Read the model definition and answer for the solid it produces. Units are mm, in the model's axes. Face numbers are marked on the shaded views. A direction names the side the tool comes from. Round coordinates to 2 decimals unless told otherwise and drop trailing zeros. Write each loop counter-clockwise with the first axis right and the second up, starting at its lowest first coordinate (ties: lowest second). Pieces come first, ordered by that corner, then holes.
Autodesk Fusion 360 part; units mm, degrees
sketch "Sketch1" plane through (0, 0, 0) normal (0, 0, 1) x (1, 0, 0)
  line L0 (0, 3) -> (10.5, 3)
  line L1 (10.5, 3) -> (10.5, 0)
  line L2 (10.5, 0) -> (0, 0)
  line L3 (0, 6) -> (13.5, 6)
  line L4 (13.5, 6) -> (13.5, 0)
  line L5 (13.5, 0) -> (18.5, 0)
  line L6 (18.5, 0) -> (18.5, -3)
  line L7 (18.5, -3) -> (0, -3)
  line L8 (0, 6) -> (0, 3)
  line L9 (0, -3) -> (0, 0)
  dimension "d1" = 10.5
  dimension "d2" = 3
  dimension "d3" = 3
  dimension "d4" = 6
  dimension "d5" = 3
  dimension "d6" = 5
extrude "Extrude1" add sketch "Sketch1" along normal blind 20
fillet "Fillet1" radius 1 2 edges at (10.5, 3, 10) (10.5, 0, 10)
fillet "Fillet1" radius 3 2 edges at (13.5, 6, 10) (13.5, 0, 10)
fillet "Fillet1" radius 1 1 edges at (18.5, 0, 10)
mirror "Mirror1" about plane through (0, -3, 0) normal (-1, 0, 0) of bodies 1 merged
chamfer "Chamfer1" distance 0.6 angle 45 2 faces at (-3.1667, -2, 20) (-3.1667, -2, 0)
chamfer "Chamfer1" distance 0.6 angle 45 2 edges at (18.5, -3, 10) (-18.5, -3, 10)
sketch "Sketch2" plane through (0, 6, 0) normal (0, 1, 0) x (-1, 0, 0)
  line L0 (10.5, 19.4) -> (-10.5, 19.4)
  line L1 (-10.5, 19.4) -> (-10.5, 0.6)
  line L2 (-10.5, 0.6) -> (10.5, 0.6)
  line L3 (10.5, 0.6) -> (10.5, 19.4)
  line L4 (-10.5, 0.6) -> (10.5, 19.4) construction
  line L5 (-6.0622, 13.5) -> (-6.0622, 6.5)
  line L6 (-6.0622, 6.5) -> (0, 3)
  line L7 (0, 3) -> (6.0622, 6.5)
  line L8 (6.0622, 6.5) -> (6.0622, 13.5)
  line L9 (6.0622, 13.5) -> (0, 17)
  line L10 (0, 17) -> (-6.0622, 13.5)
  point P0 (0, 10)
  point P1 (0, 10)
  dimension "d19" = 7
extrude "Extrude2" cut sketch "Sketch2" against normal up to surface (3 mm away) contours L5 L6 L7 L8 L9 L10
chamfer "Chamfer2" distance 0.6 angle 45 12 edges at (-3.0311, 6, 4.75) (-6.0622, 6, 10) (-3.0311, 6, 15.25) (3.0311, 6, 15.25) (6.0622, 6, 10) (3.0311, 6, 4.75) (-3.0311, 3, 4.75) (3.0311, 3, 4.75) (6.0622, 3, 10) (3.0311, 3, 15.25) (-3.0311, 3, 15.25) (-6.0622, 3, 10)
hole "Hole1" at (0, 0, 10) direction (0, -1, 0) diameter 3.3 depth 2.8 tip angle 180 countersink diameter 5.5 countersink angle 90
equation "d1 = ( 21 / 2 ) * 1 mm"
equation "d3 = d2"
equation "d4 = 2 * d2"
equation "d5 = d2"
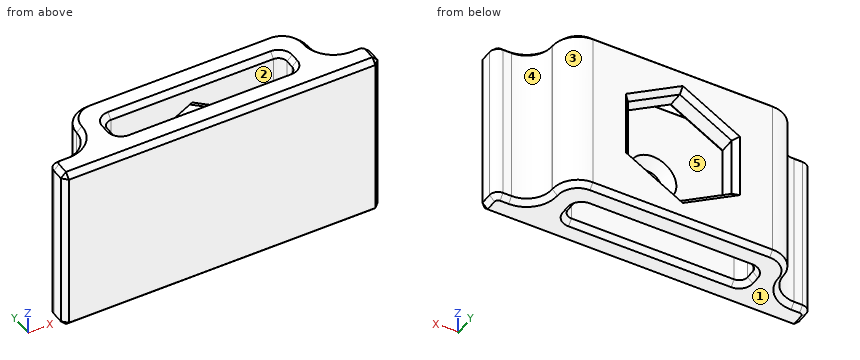
Q1. Section A-A (x = 8) is taken. Determine the outline of the cut face in (y, z), then the cut area to 3 significant figures.
Verdict:
outline: (-3, 0.6) - (-2.4, 0) - (-0.6, 0) - (0, 0.6) - (0, 19.4) - (-0.6, 20) - (-2.4, 20) - (-3, 19.4) - close; (3, 0.6) - (3.6, 0) - (5.4, 0) - (6, 0.6) - (6, 19.4) - (5.4, 20) - (3.6, 20) - (3, 19.4) - close
area: 119 mm2
Q2. Straight lines are drawn through the part: probe 1 along Y at (x, z) = (5, 16); probe 2 along Z at (x, y) = (0, -1.45); probe 3 along X at (y, z) = (-1.75, 10). For each, find the intervals that lie inside material, in ascending order.
Verdict:
probe 1: y = -3 to 0, 3 to 6
probe 2: z = 0 to 8.35, 11.65 to 20
probe 3: x = -18.5 to -1.65, 1.65 to 18.5
Q3. Determine the mould class of the marked faces 1, 2 and 3 for opening direction X: pulls with the +X half, pulls with the -X half, needs draft (parallel to the pull), parting line crosses it, or undercut.
Verdict:
face 1: needs draft
face 2: undercut
face 3: pulls with the +X half
Q4. Which of the six approach directions +Z, -Z, +X, -X, +Y, -Y give full straight-line access (tool end or side, diameter ignored) to the marked faces 4 and 5?
Verdict:
face 4: +Z, -Z, +X, +Y
face 5: +Z, -Z
Q5. Flat-ended cylindrical pins translate along their axes: pin 1 Ø0.5 at (y, z) = (1.5, 11.5) entering from -X; pin 2 Ø0.5 at (y, z) = (5, 8.5) entering from -X; pin 3 Ø2.5 at (x, z) = (-0.5, 11) entering from +Y. Find the tip coordinate at first contact, or state that the pin passes through.
Verdict:
pin 1: stops at x = -14.06
pin 2: stops at x = -12.94
pin 3: stops at y = -0.38
